Autodesk Inventor part; units mm, degrees
ref_plane "YZ Plane" through (0, 0, 0) normal (1, 0, 0) x (0, 1, 0)
ref_plane "XZ Plane" through (0, 0, 0) normal (0, 1, 0) x (-1, 0, 0)
ref_plane "XY Plane" through (0, 0, 0) normal (0, 0, 1) x (1, 0, 0)
sketch "Sketch6" plane through (0, 0, 0) normal (0, 1, 0) x (-1, 0, 0)
  line L0 (0, 0) -> (-60.1073, 0)
  line L1 (-60.1073, 0) -> (-60.1073, 2980)
  line L2 (-60.1073, 2980) -> (0, 2980)
  line L3 (0, 2980) -> (0, 0)
  dimension "d26" = 60.1073
  dimension "d27" = 2980
extrude "Plate4" add sketch "Sketch6" along normal blind 3
sketch "Sketch9" plane through (0, 3, 0) normal (0, 1, 0) x (1, 0, 0)
  line L0 (0, -2980) -> (0, 0)
  line L1 (60.1073, -2980) -> (0, -2980)
  line L2 (60.1073, 0) -> (60.1073, -2980)
  line L3 (0, 0) -> (60.1073, 0)
  line L4 (25, -2762.0797) -> (10, -2762.0797) construction
  line L5 (10, -2762.0797) -> (10, -2562.0797) construction
  line L6 (10, -2562.0797) -> (25, -2562.0797) construction
  line L7 (25, -2562.0797) -> (25, -2762.0797) construction
  dimension "d44" = 200
  dimension "d45" = 15
  dimension "d47" = 10
mark "Mark1"
sketch "Sketch7" plane through (0, 0, 0) normal (0, -1, 0) x (1, 0, 0)
  line L0 (0, 2980) -> (60.1073, 2980)
  line L1 (0, 0) -> (0, 2980)
  line L2 (60.1073, 0) -> (0, 0)
  line L3 (60.1073, 2980) -> (60.1073, 0)
  line L4 (0, 2798) -> (31.0536, 2798)
  line L5 (31.0536, 2798) -> (31.0536, 2794.8)
  line L6 (31.0536, 2794.8) -> (0, 2794.8)
  line L7 (0, 2794.8) -> (0, 2798)
  point P0 (0, 2794.8)
  point P1 (0, 200)
  point P2 (46.4173, 200)
  point P3 (0, 2794.8)
  dimension "d29" = 31.0536
  dimension "d30" = 3.2
  dimension "d51" = 182
extrude "Extrusion2" cut sketch "Sketch7" against normal through all contours L4 L5 L6 L1
pattern_linear "Rectangular Pattern1" count 6 spacing 500 along (0, 0, -1) of "Extrusion2"
sketch "Sketch8" plane through (0, 0, 0) normal (0, -1, 0) x (1, 0, 0)
  line L0 (0, 2798) -> (31.0536, 2798)
  line L1 (31.0536, 2798) -> (31.0536, 2794.8)
  line L2 (31.0536, 2794.8) -> (0, 2794.8)
  line L3 (0, 0) -> (0, 294.8)
  line L4 (60.1073, 0) -> (0, 0)
  line L5 (60.1073, 2980) -> (60.1073, 0)
  line L6 (0, 2980) -> (60.1073, 2980)
  circle A0 centre (0, 1490) radius 25
  line L7 (0, 2798) -> (0, 2980)
  line L8 (0, 298) -> (31.0536, 298)
  line L9 (31.0536, 298) -> (31.0536, 294.8)
  line L10 (31.0536, 294.8) -> (0, 294.8)
  line L11 (0, 2298) -> (0, 2794.8)
  line L12 (0, 2298) -> (31.0536, 2298)
  line L13 (31.0536, 2298) -> (31.0536, 2294.8)
  line L14 (31.0536, 2294.8) -> (0, 2294.8)
  line L15 (0, 1798) -> (0, 2294.8)
  line L16 (0, 1798) -> (31.0536, 1798)
  line L17 (31.0536, 1798) -> (31.0536, 1794.8)
  line L18 (31.0536, 1794.8) -> (0, 1794.8)
  line L19 (0, 1298) -> (0, 1794.8)
  line L20 (0, 1298) -> (31.0536, 1298)
  line L21 (31.0536, 1298) -> (31.0536, 1294.8)
  line L22 (31.0536, 1294.8) -> (0, 1294.8)
  line L23 (0, 798) -> (0, 1294.8)
  line L24 (0, 798) -> (31.0536, 798)
  line L25 (31.0536, 798) -> (31.0536, 794.8)
  line L26 (31.0536, 794.8) -> (0, 794.8)
  line L27 (0, 298) -> (0, 794.8)
  dimension "d37" = 50
  dimension "d38" = 1490
extrude "Extrusion3" cut sketch "Sketch8" against normal through all contours L19 A0 | A0 L19
pattern_linear "Rectangular Pattern2" count 2 spacing 1480 along (0, 0, 1) of "Extrusion3"
chamfer "Corner Chamfer1" distance 6 angle 45 2 edges at (22.9129, 1.5, 2980) (60.1073, 1.5, 2980)
equation "\"d26\" = Stringer4_deep"
equation "\"d28\" = Thickness"
equation "\"BendReliefWidth\" = Thickness"
equation "\"BendReliefDepth\" = 0.5 * Thickness"
equation "\"CornerReliefSize\" = 4 * Thickness"
equation "\"MinimumRemnant\" = 2 * Thickness"
equation "\"TransitionRadius\" = BendRadius"
equation "\"JacobiRadiusSize\" = BendRadius"
equation "\"GapSize\" = Thickness"
properties part number "BSH 0361 stringer board 4" material "09g2s"
Work out the finished part from the listing and answer in its coordinate system (mm). Round coordinates to 2 decimals unless told otherwise and drop trailing zeros. Loops run counter-clockwise (first coordinate to the right, second up) from the corner with the lowest first, then second, coordinate; pieces in that order, holes last. Notation, with made-up numbers: M -21,-21.75 L 29,-21.75 A29 cw 29,13.25 Z; hole C 16.5,-3 d3. An arc over 180 degrees is marked long. Use CSV: the item, a comma, the result in double quotes.
Q1. Consider L1, parallel to Z at x = 54.5, y = 1.95; L2, parallel to Z at x = 57.5, y = 1.65. Determine where each line is inside the solid, lowest interval first.
Determined:
L1,"0 to 2979.61"
L2,"0 to 2976.61"
Q2. Section A-A, the plane z = 1490 is taken. Determine the outline of the cut face in (x, y).
Determined:
outline,"M 25,0 L 60.11,0 L 60.11,3 L 25,3 Z"
Q3. Each of these flat-tipped pins is pushed along its axis until it touches: pin 1 (1.5 mm diameter, centred on x = 10.5, y = 1.5, fed in from -Z); pin 2 (0.9 mm diameter, centred on x = 18.5, y = 2, fed in from +Z); pin 3 (0.9 mm diameter, centred on x = 14.5, y = 1, fed in from +Z). Where does it stop, or does it pass through?
Determined:
pin 1,"z = 0"
pin 2,"z = 2953.69"
pin 3,"z = 2949.96"
